Autodesk Inventor part; units mm, degrees
ref_plane "YZ Plane" through (0, 0, 0) normal (1, 0, 0) x (0, 1, 0)
ref_plane "XZ Plane" through (0, 0, 0) normal (0, 1, 0) x (-1, 0, 0)
ref_plane "XY Plane" through (0, 0, 0) normal (0, 0, 1) x (1, 0, 0)
sketch "Sketch1" plane through (0, 0, 0) normal (0, 1, 0) x (-1, 0, 0)
  line L0 (3.175, 0) -> (53.225, 0)
  line L1 (56.4, -3.175) -> (56.4, -53.225)
  line L2 (53.225, -56.4) -> (3.175, -56.4)
  line L3 (0, -53.225) -> (0, -3.175)
  arc A0 (56.4, -3.175) -> (53.225, 0) centre (53.225, -3.175) ccw
  arc A1 (3.175, 0) -> (0, -3.175) centre (3.175, -3.175) ccw
  arc A2 (0, -53.225) -> (3.175, -56.4) centre (3.175, -53.225) ccw
  arc A3 (53.225, -56.4) -> (56.4, -53.225) centre (53.225, -53.225) ccw
  point P0 (0, 0)
  point P1 (56.4, -56.4)
  point P2 (56.4, 0)
  point P3 (0, -56.4)
  dimension "d0" = 56.4
  dimension "d1" = 56.4
  dimension "d2" = 3.175
extrude "Extrusion1" add sketch "Sketch1" along normal blind 56
sketch "Sketch2" plane through (0, 56, 0) normal (0, 1, 0) x (1, 0, 0)
  line L0 (0, 0) -> (-56.4, 0) construction
  line L1 (-56.4, 0) -> (-56.4, 56.4) construction
  line L2 (-56.4, 56.4) -> (0, 56.4) construction
  line L3 (0, 56.4) -> (0, 0) construction
  line L4 (-56.4, 0) -> (0, 56.4) construction
  line L5 (-4.63, 4.63) -> (-51.77, 4.63) construction
  line L6 (-51.77, 4.63) -> (-51.77, 51.77) construction
  line L7 (-51.77, 51.77) -> (-4.63, 51.77) construction
  line L8 (-4.63, 51.77) -> (-4.63, 4.63) construction
  line L9 (-4.63, 4.63) -> (-51.77, 51.77) construction
  line L10 (-51.77, 4.63) -> (-4.63, 51.77) construction
  circle A0 centre (-51.8006, 4.5994) radius 2.5
  circle A1 centre (-51.77, 51.77) radius 2.5
  circle A2 centre (-4.63, 51.77) radius 2.5
  circle A3 centre (-4.63, 4.63) radius 2.5
  point P0 (-28.2, 28.2)
  dimension "d5" = 47.14
  dimension "d6" = 47.14
  dimension "d7" = 5
  dimension "d8" = 5
  dimension "d9" = 5
  dimension "d10" = 5
hole "Hole1" at (-51.77, 56, -51.77) at (-4.63, 56, -51.77) at (-51.77, 56, -4.63) at (-4.63, 56, -4.63) direction (0, -1, 0) diameter 2.4638 depth 12 tip angle 118
sketch "Sketch3" plane through (0, 56, 0) normal (0, 1, 0) x (1, 0, 0)
  line L0 (0, 0) -> (-56.4, 56.4) construction
  circle A0 centre (-28.2, 28.2) radius 19.05
  dimension "d18" = 38.1
extrude "Extrusion2" add sketch "Sketch3" along normal blind 1.6
sketch "Sketch4" plane through (-28.2, 57.6, -28.2) normal (0, 1, 0) x (1, 0, 0)
  circle A0 centre (0, 0) radius 3.175
  point P0 (28.2, -28.2)
  dimension "d21" = 6.35
extrude "Extrusion3" add sketch "Sketch4" along normal blind 21
properties part number "NEMA23 Motor"
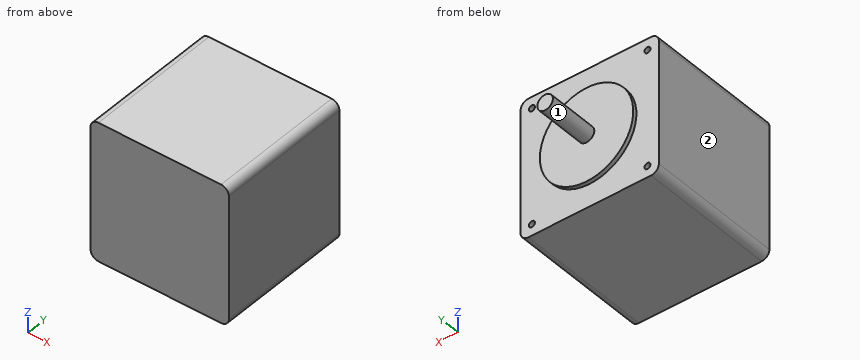
Work out the finished part from the listing and answer in its coordinate system (mm). Face numbers are marked on the shaded views. A direction names the side the tool comes from. Round coordinates to 2 decimals unless told otherwise and drop trailing zeros. Order: outer loops, then holes, each group sorted by start corner. A loop starts at its lowest first (then second) coordinate and runs counter-clockwise, first axis right, second up. Notation, with made-up numbers: M -16.75,74 L 29.25,74 A23 cw 29.25,96 Z; hole C -2,64 d11. An arc over 180 degrees is marked long. Put each result on its own line as item: value. Start each with the question number.
Q1. Flat-ended cylindrical pins translate along their axes: pin 1 (2 mm diameter, centred on x = -6, z = -15, fed in from +Y); pin 2 (3 mm diameter, centred on x = -47.5, z = -26, fed in from +Y). Find the tip coordinate at first contact, or state that the pin passes through.
Q2. Section B-B, the plane x = -16.5 is taken. Write down the section's boundary in (y, z).
Q3. Section A-A, the plane z = -28.2 is taken. Write down the section's boundary in (x, y) (3 decimals).
Q4. Section D-D, the plane x = -29 is taken. Write down the section's boundary in (y, z).
Q5. A tool of negligible diameter and unlimited length cuts with its end or side. For the marked faces 1 and 2, from which of +Z, -Z, +X, -X, +Y, -Y can it reach the whole face along a straight path? Write none if from no direction.
Q6. Straight lines are drawn through the part: L1, parallel to X at y = 49.25, z = -4.63; L2, parallel to X at y = 49, z = -4. For each, find the intervals that lie inside material, in ascending order. Write a range as [from, to].
Q7. Section C-C, the plane y = 62 is taken. Write down the section's boundary in (x, z) (3 decimals).
Findings below:
1. pin 1: stops at y = 56
1. pin 2: stops at y = 57.6
2. outline: M 0,-56.4 L 56,-56.4 L 56,-43.23 L 57.6,-43.23 L 57.6,-13.17 L 56,-13.17 L 56,0 L 0,0 Z
3. outline: M -56.4,0 L 0,0 L 0,56 L -9.15,56 L -9.15,57.6 L -25.025,57.6 L -25.025,78.6 L -31.375,78.6 L -31.375,57.6 L -47.25,57.6 L -47.25,56 L -56.4,56 Z
4. outline: M 0,-56.4 L 56,-56.4 L 56,-47.23 L 57.6,-47.23 L 57.6,-31.27 L 78.6,-31.27 L 78.6,-25.13 L 57.6,-25.13 L 57.6,-9.17 L 56,-9.17 L 56,0 L 0,0 Z
5. face 1: +Y
5. face 2: +Z, -Z, -X, +Y, -Y
6. L1: x = [-56.4, -53], [-50.54, -5.86], [-3.4, 0]
6. L2: x = [-56.4, -52.83], [-50.71, -5.69], [-3.57, 0]
7. outline: C -28.2,-28.2 d6.35
